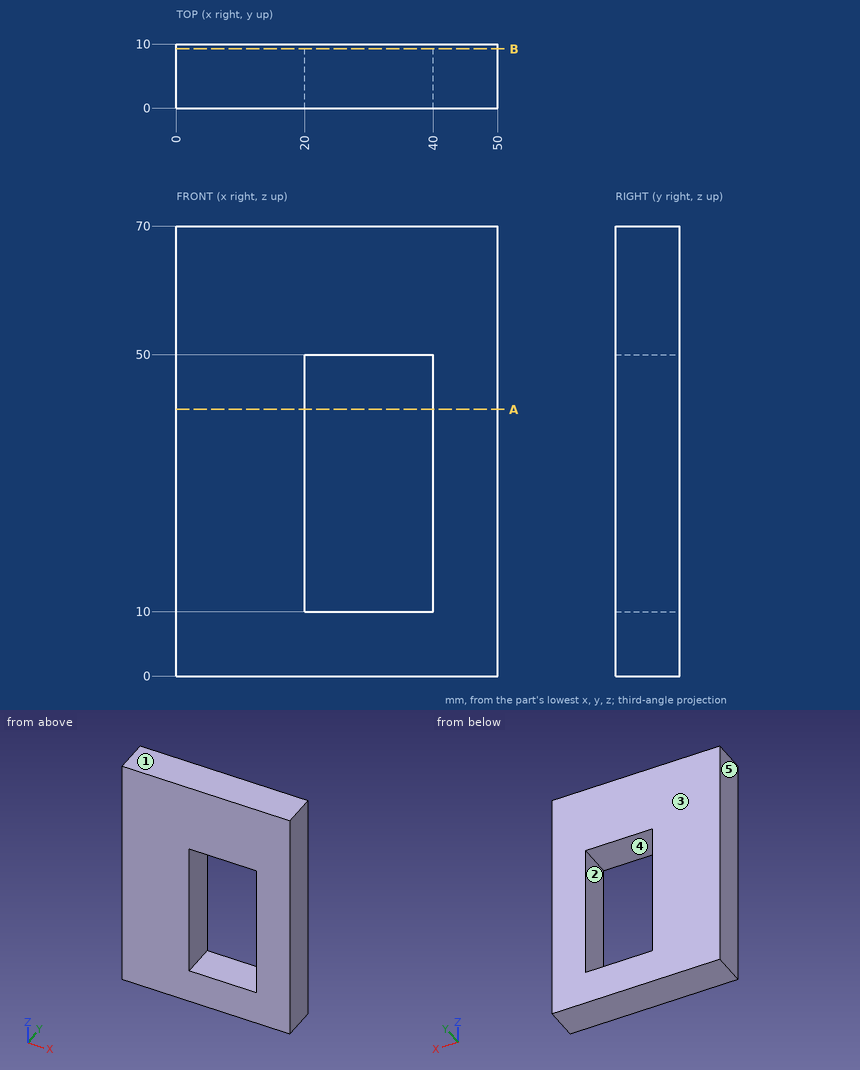
Job drawing, mm, ordinate dimensions from the low corner. One solid piece. A direction names the side the tool comes from. Round coordinates to 2 decimals unless told otherwise and drop trailing zeros. Loops run counter-clockwise (first coordinate to the right, second up) from the corner with the lowest first, then second, coordinate; pieces in that order, holes last. Notation, with made-up numbers: (-0.5, -20) -> (30.5, -20) arc R14 cw to (30.5, 3) -> close; hole circle Ø3 at (13, -28). An arc over 180 degrees is marked (long way). One line per item, written item: value. Start each with the question number.
Q1. Probe line 1 along Z through (x, y) = (36, 7); line 2 along X through (y, z) = (8, 36.5). List the from-to ranges inside material, lowest first.
Q2. Two-plate mould, pull along Z, no slides. Class the marked faces 1, 2 and 3: released by +Z, released by -Z, zero draft, split by the parting line, or undercut.
Q3. Cut at B-B on y = 9.25. List the corners of the cut face in (x, z).
Q4. Cut at A-A on z = 41.5. List the corners of the cut face in (x, y), plus the area to 3 significant figures.
Q5. 3-axis set-ups, long thin cutter, end or side, ignore diameter. For the marked faces 4 and 5: which of +Z, -Z, +X, -X, +Y, -Y reach the whole face in a straight line?
Computed:
1. line 1: 0 to 10, 50 to 70
1. line 2: 0 to 20, 40 to 50
2. face 1: released by +Z
2. face 2: undercut
2. face 3: zero draft
3. outline: (0, 0) -> (50, 0) -> (50, 70) -> (0, 70) -> close; hole (20, 10) -> (40, 10) -> (40, 50) -> (20, 50) -> close
4. outline: (0, 0) -> (20, 0) -> (20, 10) -> (0, 10) -> close; (40, 0) -> (50, 0) -> (50, 10) -> (40, 10) -> close
4. area: 300 mm²
5. face 4: +Y, -Y
5. face 5: +Z, -Z, -X, +Y, -Y
